For this review, take the finished solid that the model builds, in its own axes (mm). A direction names the side the tool comes from. Coordinates: 2 decimals unless noted, no trailing zeros. Order: outer loops, then holes, each group sorted by start corner. A loop starts at its lowest first (then second) coordinate and runs counter-clockwise, first axis right, second up. Notation, with made-up numbers: (-4.5, 61.5) -> (38.5, 61.5) arc R31 cw to (38.5, 93.5) -> close; hole circle Ø10 at (-27, 27). An arc over 180 degrees is marked (long way). Return JSON: item names as keys, results as strings. Group by question number.
Item 1: Take a section at C-C (z = -10). Write out the cut boundary in (x, y), then the cut area to 3 significant figures.
Item 2: Insertion check: pin 1 (1.5 mm diameter, centred on x = -12, y = -2, fed in from -Z); pin 2 (4 mm diameter, centred on x = 20.58, y = -7.6, fed in from +Z); pin 3 (12 mm diameter, centred on x = -4.5, z = 11, fed in from -Y). Each pin has a flat end and moves straight along its axis. Give the tip position at first contact, or say it passes through.
Item 3: For line 1 along Z through (x, y) = (-2.5, -11); line 2 along Z through (x, y) = (-2, -1.5); line 3 along Y through (x, z) = (22.5, 18.5), list the stretches that pass through material, from the lowest coordinate up.
Item 4: Take a section at A-A (x = 0). Count the separate pieces of the cut face and the enclosed holes in it, then the cut area to 3 significant figures.
Item 5: Machinability: for faces 5 (the cylindrical face through (18.777, -8.983, 24.595)), 6 (the flat face through (0, -11, -23.812)), which of the approach directions +Z, -Z, +X, -X, +Y, -Y give a long, thin tool a straight path to every point of the face, cutting with its end or side? Answer none if there is none.
Item 6: Draft analysis for pull direction Y (two halves, no side actions). For faces 1 (the flat face through (0, -11, 23.812)), 2 (the cylindrical face through (0.444, -0.161, -24.495)), 3 (the cylindrical face through (0.44, -1.75, 22.91)), 4 (the cylindrical face through (18.777, -8.983, -24.595)), state which applies: +Y half, -Y half, draft (parallel to the pull), parting line (faces both ways), or undercut.
```python
from build123d import *

# Parameters (mm, degrees)
F1_DEPTH      = 31.75
F2_R          = 2.2595381717
F2_R_2        = 2.4154540774
F2_R_3        = 2.2678572685
F3_DEPTH      = 25.401
F3_DEPTH_BACK = 25.401


with BuildPart() as f1:
    # F0 (on Right) → F1 (new body, symmetric)
    with BuildSketch(Plane.YZ):
        with BuildLine():
            Line((-0.79375, 0), (0.79375, 0))
            Line((0.79375, 0), (0.79375, 22.225))
            ThreePointArc((0.79375, 22.225), (-0.1361859697, 24.4700640303), (-2.38125, 25.4))
            Line((-2.38125, 25.4), (-11.90625, 25.4))
            Line((-11.90625, 25.4), (-11.90625, 23.8125))
            Line((-11.90625, 23.8125), (-3.96875, 23.8125))
            ThreePointArc((-3.96875, 23.8125), (-1.7236859697, 22.8825640303), (-0.79375, 20.6375))
            Line((-0.79375, 20.6375), (-0.79375, 0))
        make_face()
        with BuildLine():
            Line((0.79375, -22.225), (0.79375, 0))
            Line((0.79375, 0), (-0.79375, 0))
            Line((-0.79375, 0), (-0.79375, -20.6375))
            ThreePointArc((-0.79375, -20.6375), (-1.7236859697, -22.8825640303), (-3.96875, -23.8125))
            Line((-3.96875, -23.8125), (-11.90625, -23.8125))
            Line((-11.90625, -23.8125), (-11.90625, -25.4))
            Line((-11.90625, -25.4), (-2.38125, -25.4))
            ThreePointArc((-2.38125, -25.4), (-0.1361859697, -24.4700640303), (0.79375, -22.225))
        make_face()
    extrude(amount=F1_DEPTH, both=True)

    # F2 (on Top) → F3 (cut, two sides)
    with BuildSketch(Plane.XY) as f3_sk:
        with Locations((0, -7.6030581258)):
            Circle(F2_R)
        with Locations((-18.9749002457, -7.6030581258)):
            Circle(F2_R_2)
        with Locations((20.5765273422, -7.6030581258)):
            Circle(F2_R_3)
    extrude(amount=-F3_DEPTH, mode=Mode.SUBTRACT)
    extrude(f3_sk.sketch, amount=F3_DEPTH_BACK, mode=Mode.SUBTRACT)


solid = f1.part
```
Findings below:
{
 "1": {"outline": "(-31.75, -0.79) -> (31.75, -0.79) -> (31.75, 0.79) -> (-31.75, 0.79) -> close", "area": "101 mm2"},
 "2": {"pin 1": "stops at z = -25.4", "pin 2": "passes through", "pin 3": "stops at y = -0.79"},
 "3": {"line 1": "z = -25.4 to -23.81, 23.81 to 25.4", "line 2": "z = -25.28 to -22.63, 22.63 to 25.28", "line 3": "y = -0.79 to 0.79"},
 "4": {"separate pieces": "3", "enclosed holes": "0", "area": "102 mm2"},
 "5": {"face 5": "+Z, -Z", "face 6": "+X, -X, -Y"},
 "6": {"face 1": "draft", "face 2": "+Y half", "face 3": "-Y half", "face 4": "undercut"}
}
